Here's how the part is built. I have some questions about the finished solid (model axes, mm). Round coordinates to 2 decimals unless told otherwise and drop trailing zeros. Loops run counter-clockwise (first coordinate to the right, second up) from the corner with the lowest first, then second, coordinate; pieces in that order, holes last. Notation, with made-up numbers: (7.5, 62.25) - (17.5, 62.25) arc R21 cw to (17.5, 89.25) - close; hole circle Ø9 at (11, 23). An arc over 180 degrees is marked (long way). Answer as a JSON object with one key per item and string values. Group by question number.
1) Will these pins go through, and if not, where does the flat tip stop? P1, Ø1.6, axis at x = -57.28, z = -13.5, coming from the +Y side; P2, Ø1, axis at x = 20.5, y = 1.5, coming from the -Z side; P3, Ø1, axis at x = -19, y = 1, coming from the +Z side; P4, Ø0.6, axis at x = 24.5, y = 1, coming from the -Z side.
2) I want a section at B-B, the plane y = 1.4. Give the number of separate pieces and of enclosed holes in the cut face, then the cut area to 3 significant figures.
3) I want a section at C-C, the plane z = 59.5. Please give me the cut outline in (x, y).
4) I want a section at A-A, the plane z = -30. Please give me the cut outline in (x, y), then the cut area to 3 significant figures.
5) If I drill on line 1 along X through (y, z) = (1.05, -13.5); line 2 along Z through (x, y) = (32.5, 1.25); line 3 along Z through (x, y) = (45, 1.95), over which ranges is the centre line in solid material (lowest first)? Write a range as [from, to].
from build123d import *

# Parameters (mm, degrees)
SKETCH1_R           = 1.3
BOSS_EXTRUDE1_DEPTH = 2
SKETCH2_W           = 15
SKETCH2_H           = 22
CUT_EXTRUDE1_DEPTH  = 2
FILLET1_R           = 1
CUT_EXTRUDE2_DEPTH  = 2
SKETCH5_R           = 1.65
CUT_EXTRUDE3_DEPTH  = 2


with BuildPart() as part:
    # Sketch1 → Boss-Extrude1 (new body)
    with BuildSketch(Plane(origin=(0, 0, 0), x_dir=(1, 0, 0), z_dir=(0, 1, 0))):
        Polygon((0, -80), (69.282032303, -40), (69.282032303, 40), (0, 80), (-69.282032303, 40), (-69.282032303, -40), align=None)
        with Locations(Location((65.282032303, 13.5, 0), (0, 0, 270))):
            Circle(SKETCH1_R, mode=Mode.SUBTRACT)
        with Locations(Location((57.282032303, 13.5, 0), (0, 0, 270))):
            Circle(SKETCH1_R, mode=Mode.SUBTRACT)
        with Locations(Location((51.782032303, 8, 0), (0, 0, 270))):
            Circle(SKETCH1_R, mode=Mode.SUBTRACT)
        with Locations(Location((51.782032303, -8, 0), (0, 0, 270))):
            Circle(SKETCH1_R, mode=Mode.SUBTRACT)
        with Locations(Location((57.282032303, -13.5, 0), (0, 0, 270))):
            Circle(SKETCH1_R, mode=Mode.SUBTRACT)
        with Locations(Location((65.282032303, -13.5, 0), (0, 0, 270))):
            Circle(SKETCH1_R, mode=Mode.SUBTRACT)
        with Locations(Location((32.819219382, -40.844555434, 0), (0, 0, 270))):
            Circle(SKETCH1_R, mode=Mode.SUBTRACT)
        with Locations(Location((20.9496732, -63.285898385, 0), (0, 0, 270))):
            Circle(SKETCH1_R, mode=Mode.SUBTRACT)
        with Locations(Location((16.9496732, -56.357695155, 0), (0, 0, 270))):
            Circle(SKETCH1_R, mode=Mode.SUBTRACT)
        with Locations(Location((18.962812921, -48.844555434, 0), (0, 0, 270))):
            Circle(SKETCH1_R, mode=Mode.SUBTRACT)
        with Locations(Location((44.332359102, -49.785898385, 0), (0, 0, 270))):
            Circle(SKETCH1_R, mode=Mode.SUBTRACT)
        with Locations(Location((40.332359102, -42.857695155, 0), (0, 0, 270))):
            Circle(SKETCH1_R, mode=Mode.SUBTRACT)
        with Locations(Location((-44.332359102, -49.785898385, 0), (0, 0, 270))):
            Circle(SKETCH1_R, mode=Mode.SUBTRACT)
        with Locations(Location((-40.332359102, -42.857695155, 0), (0, 0, 270))):
            Circle(SKETCH1_R, mode=Mode.SUBTRACT)
        with Locations(Location((-32.819219382, -40.844555434, 0), (0, 0, 270))):
            Circle(SKETCH1_R, mode=Mode.SUBTRACT)
        with Locations(Location((-18.962812921, -48.844555434, 0), (0, 0, 270))):
            Circle(SKETCH1_R, mode=Mode.SUBTRACT)
        with Locations(Location((-16.9496732, -56.357695155, 0), (0, 0, 270))):
            Circle(SKETCH1_R, mode=Mode.SUBTRACT)
        with Locations(Location((-20.9496732, -63.285898385, 0), (0, 0, 270))):
            Circle(SKETCH1_R, mode=Mode.SUBTRACT)
        with Locations(Location((18.962812921, 48.844555434, 0), (0, 0, 270))):
            Circle(SKETCH1_R, mode=Mode.SUBTRACT)
        with Locations(Location((44.332359102, 49.785898385, 0), (0, 0, 270))):
            Circle(SKETCH1_R, mode=Mode.SUBTRACT)
        with Locations(Location((40.332359102, 42.857695155, 0), (0, 0, 270))):
            Circle(SKETCH1_R, mode=Mode.SUBTRACT)
        with Locations(Location((32.819219382, 40.844555434, 0), (0, 0, 270))):
            Circle(SKETCH1_R, mode=Mode.SUBTRACT)
        with Locations(Location((20.9496732, 63.285898385, 0), (0, 0, 270))):
            Circle(SKETCH1_R, mode=Mode.SUBTRACT)
        with Locations(Location((16.9496732, 56.357695155, 0), (0, 0, 270))):
            Circle(SKETCH1_R, mode=Mode.SUBTRACT)
        with Locations(Location((-65.282032303, 13.5, 0), (0, 0, 270))):
            Circle(SKETCH1_R, mode=Mode.SUBTRACT)
        with Locations(Location((-20.9496732, 63.285898385, 0), (0, 0, 270))):
            Circle(SKETCH1_R, mode=Mode.SUBTRACT)
        with Locations(Location((-16.9496732, 56.357695155, 0), (0, 0, 270))):
            Circle(SKETCH1_R, mode=Mode.SUBTRACT)
        with Locations(Location((-18.962812921, 48.844555434, 0), (0, 0, 270))):
            Circle(SKETCH1_R, mode=Mode.SUBTRACT)
        with Locations(Location((-32.819219382, 40.844555434, 0), (0, 0, 270))):
            Circle(SKETCH1_R, mode=Mode.SUBTRACT)
        with Locations(Location((-44.332359102, 49.785898385, 0), (0, 0, 270))):
            Circle(SKETCH1_R, mode=Mode.SUBTRACT)
        with Locations(Location((-40.332359102, 42.857695155, 0), (0, 0, 270))):
            Circle(SKETCH1_R, mode=Mode.SUBTRACT)
        with Locations(Location((-57.282032303, 13.5, 0), (0, 0, 270))):
            Circle(SKETCH1_R, mode=Mode.SUBTRACT)
        with Locations(Location((-51.782032303, 8, 0), (0, 0, 270))):
            Circle(SKETCH1_R, mode=Mode.SUBTRACT)
        with Locations(Location((-51.782032303, -8, 0), (0, 0, 270))):
            Circle(SKETCH1_R, mode=Mode.SUBTRACT)
        with Locations(Location((-57.282032303, -13.5, 0), (0, 0, 270))):
            Circle(SKETCH1_R, mode=Mode.SUBTRACT)
        with Locations(Location((-65.282032303, -13.5, 0), (0, 0, 270))):
            Circle(SKETCH1_R, mode=Mode.SUBTRACT)
    extrude(amount=BOSS_EXTRUDE1_DEPTH)

    # Sketch2 → Cut-Extrude1 (cut)
    with BuildSketch(Plane(origin=(0, 2, 0), x_dir=(1, 0, 0), z_dir=(0, 1, 0))):
        with Locations((61.782032303, 0)):
            Rectangle(SKETCH2_W, SKETCH2_H)
        Polygon((44.167295593, -54.5), (36.667295593, -41.509618943), (17.61473671, -52.509618943), (25.11473671, -65.5), align=None)
        Polygon((-25.11473671, -65.5), (-44.167295593, -54.5), (-36.667295593, -41.509618943), (-17.61473671, -52.509618943), align=None)
        Polygon((25.11473671, 65.5), (17.61473671, 52.509618943), (36.667295593, 41.509618943), (44.167295593, 54.5), align=None)
        Polygon((-44.167295593, 54.5), (-25.11473671, 65.5), (-17.61473671, 52.509618943), (-36.667295593, 41.509618943), align=None)
        with Locations((-61.782032303, 0)):
            Rectangle(SKETCH2_W, SKETCH2_H)
    extrude(amount=-CUT_EXTRUDE1_DEPTH, mode=Mode.SUBTRACT)

    # Fillet1
    fillet1_edges = [part.edges().sort_by_distance(p)[0] for p in [
        (69.282032303, 1, -11),
        (69.282032303, 1, 11),
        (44.167295593, 1, 54.5),
        (25.11473671, 1, 65.5),
        (-25.11473671, 1, 65.5),
        (-44.167295593, 1, 54.5),
        (25.11473671, 1, -65.5),
        (44.167295593, 1, -54.5),
        (-44.167295593, 1, -54.5),
        (-25.11473671, 1, -65.5),
        (-69.282032303, 1, 11),
        (-69.282032303, 1, -11),
        (-69.282032303, 1, -40),
        (0, 1, -80),
        (69.282032303, 1, -40),
        (69.282032303, 1, 40),
        (0, 1, 80),
        (-69.282032303, 1, 40),
    ]]
    fillet(fillet1_edges, radius=FILLET1_R)

    # Sketch3 → Cut-Extrude2 (cut)
    with BuildSketch(Plane(origin=(0, 2, 0), x_dir=(1, 0, 0), z_dir=(0, 1, 0))):
        with BuildLine():
            Line((-32, 32.6), (-12, 32.6))
            ThreePointArc((-12, 32.6), (-9.4, 30), (-12, 27.4))
            Line((-12, 27.4), (-32, 27.4))
            ThreePointArc((-32, 27.4), (-34.6, 30), (-32, 32.6))
        make_face()
        with BuildLine():
            Line((-32, 2.6), (-12, 2.6))
            ThreePointArc((-12, 2.6), (-9.4, 0), (-12, -2.6))
            Line((-12, -2.6), (-32, -2.6))
            ThreePointArc((-32, -2.6), (-34.6, 0), (-32, 2.6))
        make_face()
        with BuildLine():
            Line((-32, -27.4), (-12, -27.4))
            ThreePointArc((-12, -27.4), (-9.4, -30), (-12, -32.6))
            Line((-12, -32.6), (-32, -32.6))
            ThreePointArc((-32, -32.6), (-34.6, -30), (-32, -27.4))
        make_face()
        with BuildLine():
            Line((32, -32.6), (12, -32.6))
            ThreePointArc((12, -32.6), (9.4, -30), (12, -27.4))
            Line((12, -27.4), (32, -27.4))
            ThreePointArc((32, -27.4), (34.6, -30), (32, -32.6))
        make_face()
        with BuildLine():
            Line((32, 27.4), (12, 27.4))
            ThreePointArc((12, 27.4), (9.4, 30), (12, 32.6))
            Line((12, 32.6), (32, 32.6))
            ThreePointArc((32, 32.6), (34.6, 30), (32, 27.4))
        make_face()
        with BuildLine():
            Line((32, -2.6), (12, -2.6))
            ThreePointArc((12, -2.6), (9.4, 0), (12, 2.6))
            Line((12, 2.6), (32, 2.6))
            ThreePointArc((32, 2.6), (34.6, 0), (32, -2.6))
        make_face()
    extrude(amount=-CUT_EXTRUDE2_DEPTH, mode=Mode.SUBTRACT)

    # Sketch5 → Cut-Extrude3 (cut)
    with BuildSketch(Plane(origin=(0, 2, 0), x_dir=(1, 0, 0), z_dir=(0, 1, 0))):
        with Locations(Location((-26.85, 24, 0), (0, 0, 270))):
            Circle(SKETCH5_R)
        with Locations(Location((27.584263601, 24, 0), (0, 0, 270))):
            Circle(SKETCH5_R)
        with Locations(Location((26.85, -20.7, 0), (0, 0, 270))):
            Circle(SKETCH5_R)
        with Locations(Location((-26.85, -20.7, 0), (0, 0, 270))):
            Circle(SKETCH5_R)
    extrude(amount=-CUT_EXTRUDE3_DEPTH, mode=Mode.SUBTRACT)


solid = part.part
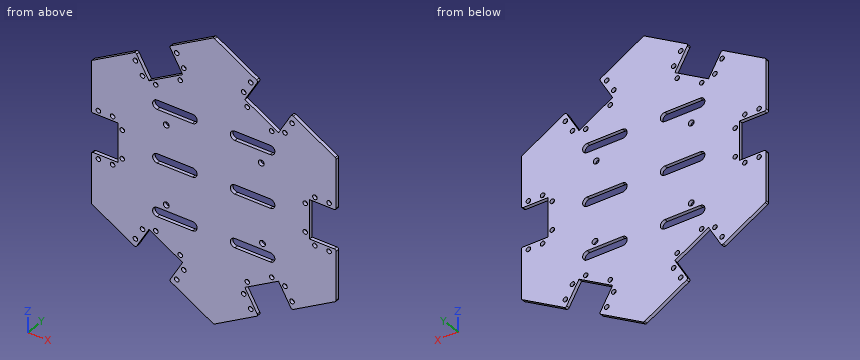
Outcome:
{
 "1": {"P1": "through", "P2": "z = -68.45", "P3": "z = 69.32", "P4": "z = -66.03"},
 "2": {"separate pieces": "1", "enclosed holes": "46", "area": "13,700 mm^2"},
 "3": {"outline": "(-21.65, 0) - (21.65, 0) - (21.65, 2) - (-21.65, 2) - close"},
 "4": {"outline": "(-69.28, 0) - (-34.6, 0) - (-34.6, 2) - (-69.28, 2) - close; (-9.4, 0) - (9.4, 0) - (9.4, 2) - (-9.4, 2) - close; (34.6, 0) - (69.28, 0) - (69.28, 2) - (34.6, 2) - close", "area": "176 mm^2"},
 "5": {"line 1": "[-69.28, -66.58], [-63.98, -58.58], [-55.98, 55.98], [58.58, 63.98], [66.58, 69.28]", "line 2": "[-43.92, -42.1], [-39.58, -32.55], [-27.45, -2.55], [2.55, 27.45], [32.55, 39.58], [42.1, 43.92]", "line 3": "[-54.02, -50.9], [-48.67, 48.67], [50.9, 54.02]"}
}
